Build history of the part. All positions in model axes, mm. Give positions to 0.01 mm unless a question says otherwise; leave off trailing zeros. Loops run counter-clockwise (first coordinate to the right, second up) from the corner with the lowest first, then second, coordinate; pieces in that order, holes last. Notation, with made-up numbers: (62, -2) -> (83, -2) arc R24 ccw to (83, 25) -> close; hole circle Ø6 at (31, 9). An arc over 180 degrees is marked (long way). Answer as a JSON object with one key per item and string values. Group by question number.
Q1. Drop flat-ended pins along their axis: pin 1 (10 mm diameter, centred on x = 32, y = 26.5, fed in from -Z); pin 2 (12 mm diameter, centred on x = -30.5, z = 21.5, fed in from +Y); pin 3 (3 mm diameter, centred on x = -15.5, z = 11, fed in from +Y); pin 4 (8 mm diameter, centred on y = 29.5, z = 6.5, fed in from -X). Give the stop position or say it passes through.
Q2. Wall check: probe 1 along Y at (x, z) = (11.5, 42.5); probe 2 along Z at (x, y) = (-5, 10.5); probe 3 along Z at (x, y) = (-39, 28). Give the ranges that are in metal, low to high. Write a range as from..to.
Q3. Band-saw the part on B-B, the plane y = 31.5. Write the cut outline in (x, z).
Q4. Band-saw the part on A-A, the plane x = -15. Write the cut outline in (y, z), plus the area to 3 significant figures.
from build123d import *

# Parameters (mm, degrees)
ESBO_O2_R                  = 45
RESSALTO_EXTRUS_O3_DEPTH   = 45
CORTE_EXTRUS_O1_DEPTH      = 136
CORTE_EXTRUS_O1_DEPTH_BACK = 136
ESBO_O5_R                  = 42
CORTE_EXTRUS_O2_DEPTH      = 136
CORTE_EXTRUS_O2_DEPTH_BACK = 136


with BuildPart() as part:
    # Esboço2 → Ressalto-extrusão3 (new, symmetric)
    with BuildSketch(Plane(origin=(0, 0, 0), x_dir=(0, 0, -1), z_dir=(1, 0, 0))):
        with Locations(Location((-45, 45, 0), (0, 0, 180))):
            Circle(ESBO_O2_R)
    extrude(amount=RESSALTO_EXTRUS_O3_DEPTH, both=True)

    # Esboço5 → Corte-extrusão1 (cut, two sides: drawn at the far end of the back side and taken through both)
    with BuildSketch(Plane(origin=(0, 0, 0), x_dir=(0, 0, -1), z_dir=(1, 0, 0)).offset(-CORTE_EXTRUS_O1_DEPTH_BACK)):
        with Locations((-45, 45)):
            Circle(ESBO_O5_R)
    extrude(amount=CORTE_EXTRUS_O1_DEPTH + CORTE_EXTRUS_O1_DEPTH_BACK, mode=Mode.SUBTRACT)

    # Esboço6 → Corte-extrusão2 (cut, two sides: drawn at the far end of the back side and taken through both)
    with BuildSketch(Plane(origin=(0, 0, 0), x_dir=(0, 0, -1), z_dir=(1, 0, 0)).offset(-CORTE_EXTRUS_O2_DEPTH_BACK)):
        Polygon((-45, 45), (-45, 0), (-90, 0), (-90, 45), (-90, 90), (-45, 90), (-3, 90), (0, 90), (0, 45), (-5.810711404, 29.893721195), align=None)
    extrude(amount=CORTE_EXTRUS_O2_DEPTH + CORTE_EXTRUS_O2_DEPTH_BACK, mode=Mode.SUBTRACT)


solid = part.part
Worked answers:
{
 "1": {"pin 1": "z = 2.07", "pin 2": "y = 15.1", "pin 3": "y = 22.56", "pin 4": "x = -45"},
 "2": {"probe 1": "0.07..3.07", "probe 2": "16.11..21.05", "probe 3": "3.33..6.59"},
 "3": {"outline": "(-45, 2.07) -> (45, 2.07) -> (45, 5.19) -> (-45, 5.19) -> close"},
 "4": {"outline": "(0, 45) arc R45 ccw to (45, 0) -> (29.95, 5.79) arc R42 cw to (3, 45) -> close", "area": "190 mm2"}
}
